The model under review builds one solid part; all positions refer to its coordinate system, in mm. Give positions to 0.01 mm unless a question says otherwise; leave off trailing zeros. Loops run counter-clockwise (first coordinate to the right, second up) from the corner with the lowest first, then second, coordinate; pieces in that order, holes last. Notation, with made-up numbers: M 75,-11 L 91,-11 A16 cw 91,-4 Z; hole C -5,71 d4. An arc over 180 degrees is marked long. Return JSON: item names as keys, results as strings. Group by question number.
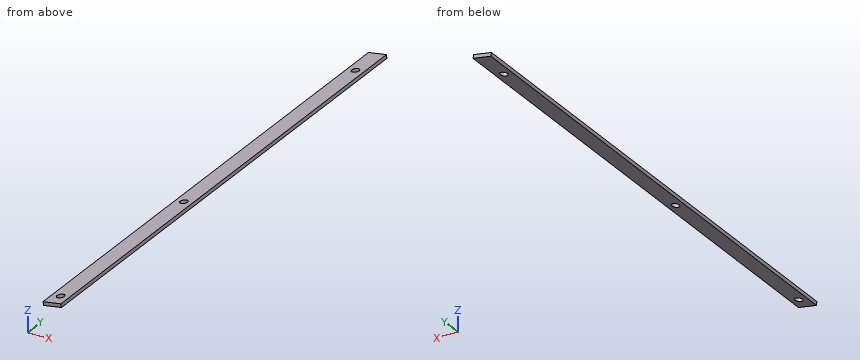
```python
from build123d import *

# Parameters (mm, degrees)
SKETCH1_W             = 8.255
SKETCH1_H             = 237.248411897
BOSS_EXTRUDE1_DEPTH   = 1.5875
CUT_EXTRUDE1_DEPTH    = 2.336885598
F_4_CLEARANCE_HOLE1_D = 3.4544


with BuildPart() as part:
    # Sketch1 → Boss-Extrude1 (new body)
    with BuildSketch(Plane(origin=(23.448725568, 0, -121.072657859), x_dir=(0.9848077530122085, 0, 0.17364817766692836), z_dir=(-0.17364817766692836, 0, 0.9848077530122085))):
        with Locations((-157.300223262, 29.663605247)):
            Rectangle(SKETCH1_W, SKETCH1_H)
    extrude(amount=BOSS_EXTRUDE1_DEPTH)

    # Sketch6 → Cut-Extrude1 (cut)
    with BuildSketch(Plane.XZ.offset(88.960600702)):
        Polygon((-135.526547851, -149.104287829), (-127.39695985, -147.670822122), (-127.672626332, -146.107439814), (-135.802214333, -147.540905521), align=None)
    extrude(amount=-CUT_EXTRUDE1_DEPTH, mode=Mode.SUBTRACT)

    # #4 Clearance Hole1 (through all)
    with Locations(Plane(origin=(21.136043007, 0, -119.868456446), x_dir=(0.9848077530122086, 0, 0.17364817766692783), z_dir=(-0.1736481776669278, 0, 0.9848077530122085))):
        with Locations((-155.231782926, -80.273715104), (-155.231782926, 132.412811195), (-155.231782926, 8.587811195)):
            Hole(F_4_CLEARANCE_HOLE1_D / 2)


solid = part.part
```
(1) Add section A-A (y = 97). Write out the cut boundary in (x, z), and give its area (3 significant figures).
(2) For probe 1 along Y at (x, z) = (-131.75, -147.7); probe 2 along Y at (x, z) = (-130, -147.9); probe 3 along Z at (x, y) = (-131.5, 78), list the stretches that pass through material, from the lowest coordinate up.
(3) For pin 1 (4 mm diameter, centred on x = -130.5, y = 113.5, fed in from +Z); pin 2 (1.5 mm diameter, centred on x = -131, y = 66.5, fed in from -Z), all flat-tipped, find the tip position at first contact; note any pin that passes through.
(4) Add section B-B (x = -131.5). Count the separate pieces of the cut face and the enclosed holes in it, and give its area (3 significant figures).
Verdict:
{
 "1": {"outline": "M -135.8,-147.54 L -135.53,-149.1 L -127.4,-147.67 L -127.67,-146.11 Z", "area": "13.1 mm²"},
 "2": {"probe 1": "y = -86.62 to -81.99, -78.55 to 6.87, 10.31 to 130.69, 134.13 to 148.29", "probe 2": "y = -86.62 to -81.09, -79.46 to 7.78, 9.4 to 131.6, 133.23 to 148.29", "probe 3": "z = -148.39 to -146.78"},
 "3": {"pin 1": "stops at z = -146.25", "pin 2": "stops at z = -148.44"},
 "4": {"separate pieces": "4", "enclosed holes": "0", "area": "362 mm²"}
}
